```python
from build123d import *

# Parameters (mm, degrees)
RIM_BARREL_START  = -14
PROFILE_1_R       = 27.5
PROFILE_1_R_2     = 24.5
RIM_BARREL_DEPTH  = 28
SPOKE_WEB_START   = 6
PROFILE_2_R       = 25
PROFILE_2_R_2     = 2.25
PROFILE_2_R_3     = 5.5
SPOKE_WEB_DEPTH   = 3
PROFILE_3_R       = 9
AF12_SOCKET_DEPTH = 6


with BuildPart() as part:
    # Profile_1 → Rim_barrel (new body)
    with BuildSketch(Plane.XY.offset(RIM_BARREL_START)):
        Circle(PROFILE_1_R)
        Circle(PROFILE_1_R_2, mode=Mode.SUBTRACT)
    extrude(amount=RIM_BARREL_DEPTH)

    # Profile_2 → Spoke_web (add)
    with BuildSketch(Plane.XY.offset(SPOKE_WEB_START)):
        Circle(PROFILE_2_R)
        Circle(PROFILE_2_R_2, mode=Mode.SUBTRACT)
        with Locations((16, 0)):
            Circle(PROFILE_2_R_3, mode=Mode.SUBTRACT)
        with Locations((9.97583683, 12.509303719)):
            Circle(PROFILE_2_R_3, mode=Mode.SUBTRACT)
        with Locations((-3.560334943, 15.598846595)):
            Circle(PROFILE_2_R_3, mode=Mode.SUBTRACT)
        with Locations((-14.415501886, 6.942139826)):
            Circle(PROFILE_2_R_3, mode=Mode.SUBTRACT)
        with Locations((-14.415501886, -6.942139826)):
            Circle(PROFILE_2_R_3, mode=Mode.SUBTRACT)
        with Locations((-3.560334943, -15.598846595)):
            Circle(PROFILE_2_R_3, mode=Mode.SUBTRACT)
        with Locations((9.97583683, -12.509303719)):
            Circle(PROFILE_2_R_3, mode=Mode.SUBTRACT)
    extrude(amount=SPOKE_WEB_DEPTH)

    # Profile_3 → AF12_socket (add)
    with BuildSketch(Plane.XY):
        Circle(PROFILE_3_R)
        Polygon((6.06, 3.498742631), (0, 6.997485263), (-6.06, 3.498742631), (-6.06, -3.498742631), (0, -6.997485263), (6.06, -3.498742631), align=None, mode=Mode.SUBTRACT)
    extrude(amount=AF12_SOCKET_DEPTH)


solid = part.part
```
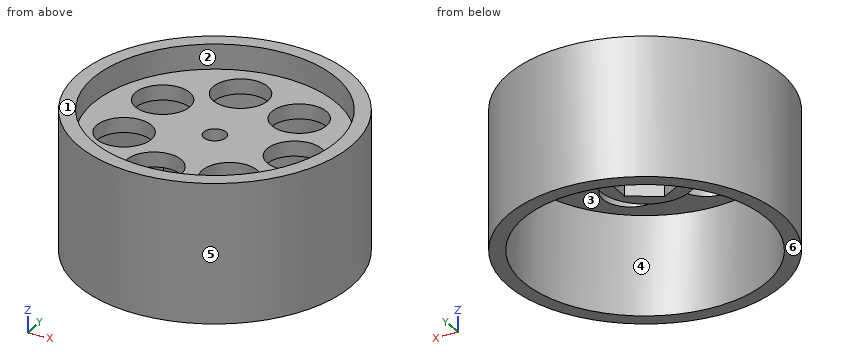
Here's how the part is built. I have some questions about the finished solid (model axes, mm). Face numbers are marked on the shaded views. A direction names the side the tool comes from. Coordinates: 2 decimals unless noted, no trailing zeros. Loops run counter-clockwise (first coordinate to the right, second up) from the corner with the lowest first, then second, coordinate; pieces in that order, holes last. Notation, with made-up numbers: (38.5, 82) -> (65.5, 82) arc R37 cw to (65.5, 120) -> close; hole circle Ø8 at (13.5, -2.5). An arc over 180 degrees is marked (long way). Return JSON: item names as keys, results as strings.
1) Will these pins go through, and if not, where does the flat tip stop? pin 1 (9.5 mm diameter, centred on x = 0, y = 2, fed in from -Z); pin 2 (14.5 mm diameter, centred on x = -3.56, y = -15.6, fed in from +Z); pin 3 (1.8 mm diameter, centred on y = -1.5, z = 2, fed in from -X).
Results below:
{"pin 1": "z = 0", "pin 2": "z = 9", "pin 3": "x = -27.49"}
2) If we section it at A-A, the plane z = 1.5: Write out the boundary of the cut face in (x, y).
Results below:
{"outline": "circle Ø55 at (0, 0); circle Ø18 at (0, 0); hole circle Ø49 at (0, 0); hole (-6.06, -3.5) -> (0, -7) -> (6.06, -3.5) -> (6.06, 3.5) -> (0, 7) -> (-6.06, 3.5) -> close"}
3) If we section it at D-D, the plane z = -6.5: Write out the boundary of the cut face in (x, y), then the cut area to 3 significant figures.
Results below:
{"outline": "circle Ø55 at (0, 0); hole circle Ø49 at (0, 0)", "area": "490 mm²"}
4) Thinking about a two-plate mould opening in Y: for the marked faces 4, 5 and 6, which applies, +Y half, -Y half, draft (parallel to the pull), parting line (faces both ways), or undercut?
Results below:
{"face 4": "undercut", "face 5": "parting line", "face 6": "draft"}
5) For the marked faces 1, 2 and 3, which set-ups out of +Z, -Z, +X, -X, +Y, -Y let a thin tool reach every point of the face, with its end or its side?
Results below:
{"face 1": "+Z, +X, -X, +Y, -Y", "face 2": "+Z", "face 3": "-Z"}
6) I need wall thicknesses on line 1 (Y direction, x = -3, z = 5.25); line 2 (X direction, y = 6.5, z = 3.25); line 3 (X direction, y = -15, z = 6.5). Which ranges of each line are inside material? Lowest first, please. Write a range as from..to.
Results below:
{"line 1": "-27.34..-24.32, -8.49..-5.27, 5.27..8.49, 24.32..27.34", "line 2": "-26.72..-23.62, -6.22..-0.86, 0.86..6.22, 23.62..26.72", "line 3": "-23.05..-9.03, 1.91..5.07, 14.88..23.05"}
7) If we section it at C-C, the plane x = 20: Write out the boundary of the cut face in (y, z).
Results below:
{"outline": "(-18.87, -14) -> (-14.15, -14) -> (-14.15, 6) -> (-3.77, 6) -> (-3.77, 9) -> (-14.15, 9) -> (-14.15, 14) -> (-18.87, 14) -> close; (3.77, 6) -> (14.15, 6) -> (14.15, -14) -> (18.87, -14) -> (18.87, 14) -> (14.15, 14) -> (14.15, 9) -> (3.77, 9) -> close"}
8) If we section it at B-B, the plane y = 0: Write out the boundary of the cut face in (x, z), then the cut area to 3 significant figures.
Results below:
{"outline": "(-27.5, -14) -> (-24.5, -14) -> (-24.5, 6) -> (-9, 6) -> (-9, 0) -> (-6.06, 0) -> (-6.06, 6) -> (-2.25, 6) -> (-2.25, 9) -> (-24.5, 9) -> (-24.5, 14) -> (-27.5, 14) -> close; (2.25, 6) -> (6.06, 6) -> (6.06, 0) -> (9, 0) -> (9, 6) -> (10.5, 6) -> (10.5, 9) -> (2.25, 9) -> close; (21.5, 6) -> (24.5, 6) -> (24.5, -14) -> (27.5, -14) -> (27.5, 14) -> (24.5, 14) -> (24.5, 9) -> (21.5, 9) -> close", "area": "304 mm²"}
